Can you work these out from the model? Positions are in its coordinate system, mm. A direction names the side the tool comes from. Round coordinates to 2 decimals unless told otherwise and drop trailing zeros. Order: outer loops, then holes, each group sorted by start corner. A loop starts at its lowest first (then second) coordinate and runs counter-clockwise, first axis right, second up.
from build123d import *

# Parameters (mm, degrees)
SKETCH_1_R          = 1.5
EXTRUDE_1_DEPTH     = 3
SKETCH_2_R          = 1.5
CUT_EXTRUDE_1_DEPTH = 55.166410256
EXTRUDE_2_DEPTH     = 3
CUT_EXTRUDE_2_DEPTH = 55.166410256
CUT_EXTRUDE_3_DEPTH = 3
FILLET_1_R          = 3
EXTRUDE_3_DEPTH     = 3
FILLET_3_R          = 4
SKETCH_9_W          = 40
SKETCH_9_H          = 28
CUT_EXTRUDE_4_DEPTH = 10
FILLET_4_R          = 5
SKETCH_11_R         = 6.275308726
SKETCH_11_R_2       = 1.5
SKETCH_11_R_3       = 5.719245844
EXTRUDE_4_DEPTH     = 3
FILLET_5_R          = 30


with BuildPart() as part:
    # 草图1 → 凸台-拉伸1 (new body)
    with BuildSketch(Plane(origin=(0, 0, 0), x_dir=(1, 0, 0), z_dir=(0, 1, 0))):
        with BuildLine():
            Line((-17.5, -25), (-30, -25))
            Line((-30, -25), (-30, 25))
            Line((-30, 25), (-30, 29.606079858))
            ThreePointArc((-30, 29.606079858), (0, 25), (30, 29.606079858))
            Line((30, 29.606079858), (30, 25))
            Line((30, 25), (30, -25))
            Line((30, -25), (17.5, -25))
            Line((17.5, -25), (17.5, -45))
            Line((17.5, -45), (-17.5, -45))
            Line((-17.5, -45), (-17.5, -25))
        make_face()
        with Locations(Location((-14, -17, 0), (0, 0, 270))):
            Circle(SKETCH_1_R, mode=Mode.SUBTRACT)
        with Locations(Location((14, -17, 0), (0, 0, 90))):
            Circle(SKETCH_1_R, mode=Mode.SUBTRACT)
        with Locations(Location((-14, -28, 0), (0, 0, 270))):
            Circle(SKETCH_1_R, mode=Mode.SUBTRACT)
        with Locations(Location((14, -28, 0), (0, 0, 90))):
            Circle(SKETCH_1_R, mode=Mode.SUBTRACT)
        with BuildLine():
            Line((9.5, 20.5), (14.5, 20.5))
            ThreePointArc((14.5, 20.5), (16, 22), (14.5, 23.5))
            Line((14.5, 23.5), (9.5, 23.5))
            ThreePointArc((9.5, 23.5), (8, 22), (9.5, 20.5))
        make_face(mode=Mode.SUBTRACT)
        with BuildLine():
            Line((-2.5, 23.5), (2.5, 23.5))
            ThreePointArc((2.5, 23.5), (4, 22), (2.5, 20.5))
            Line((2.5, 20.5), (-2.5, 20.5))
            ThreePointArc((-2.5, 20.5), (-4, 22), (-2.5, 23.5))
        make_face(mode=Mode.SUBTRACT)
        with BuildLine():
            Line((-14.5, 23.5), (-9.5, 23.5))
            ThreePointArc((-9.5, 23.5), (-8, 22), (-9.5, 20.5))
            Line((-9.5, 20.5), (-14.5, 20.5))
            ThreePointArc((-14.5, 20.5), (-16, 22), (-14.5, 23.5))
        make_face(mode=Mode.SUBTRACT)
    extrude(amount=EXTRUDE_1_DEPTH)

    # 草图2 → 切除-拉伸1 (cut, through all)
    with BuildSketch(Plane(origin=(0, 3, 0), x_dir=(1, 0, 0), z_dir=(0, 1, 0))):
        with Locations(Location((-26, 19.5, 0), (0, 0, 270))):
            Circle(SKETCH_2_R)
        with Locations(Location((26, 19.5, 0), (0, 0, 90))):
            Circle(SKETCH_2_R)
        with BuildLine():
            Line((-6.4, 15.5), (-6.4, 0.5))
            ThreePointArc((-6.4, 0.5), (-10, -3.1), (-13.6, 0.5))
            Line((-13.6, 0.5), (-13.6, 15.5))
            ThreePointArc((-13.6, 15.5), (-10, 19.1), (-6.4, 15.5))
        make_face()
        with BuildLine():
            Line((6.4, 15.5), (6.4, 0.5))
            ThreePointArc((6.4, 0.5), (10, -3.1), (13.6, 0.5))
            Line((13.6, 0.5), (13.6, 15.5))
            ThreePointArc((13.6, 15.5), (10, 19.1), (6.4, 15.5))
        make_face()
    extrude(amount=-CUT_EXTRUDE_1_DEPTH, mode=Mode.SUBTRACT)

    # 草图3 → 凸台-拉伸2 (add)
    with BuildSketch(Plane(origin=(0, 3, 0), x_dir=(1, 0, 0), z_dir=(0, 1, 0))):
        Polygon((-30, -25), (-17.5, -45), (-17.5, -25), align=None)
        Polygon((17.5, -25), (17.5, -45), (30, -25), align=None)
    extrude(amount=-EXTRUDE_2_DEPTH)

    # 草图4 → 切除-拉伸2 (cut, through all)
    with BuildSketch(Plane(origin=(0, 3, 0), x_dir=(1, 0, 0), z_dir=(0, 1, 0))):
        Polygon((-30, 15), (-17.5, -45), (-30, -25), align=None)
        Polygon((17.5, -45), (30, -25), (30, 15), align=None)
    extrude(amount=-CUT_EXTRUDE_2_DEPTH, mode=Mode.SUBTRACT)

    # 草图6 → 切除-拉伸3 (cut)
    with BuildSketch(Plane(origin=(0, 3, 0), x_dir=(1, 0, 0), z_dir=(0, 1, 0))):
        Polygon((-10, -7), (10, -7), (7, -32), (-7, -32), align=None)
    extrude(amount=-CUT_EXTRUDE_3_DEPTH, mode=Mode.SUBTRACT)

    # 圆角1
    fillet_1_edges = [part.edges().sort_by_distance(p)[0] for p in [
        (10, 1.5, 7),
        (7, 1.5, 32),
        (-7, 1.5, 32),
        (-10, 1.5, 7),
    ]]
    fillet(fillet_1_edges, radius=FILLET_1_R)

    # 草图8 → 凸台-拉伸3 (add)
    with BuildSketch(Plane(origin=(0, 3, 0), x_dir=(1, 0, 0), z_dir=(0, 1, 0))):
        Polygon((-17.5, -45), (-17.083333333, -47), (17.083333333, -47), (17.5, -45), align=None)
    extrude(amount=-EXTRUDE_3_DEPTH)

    # 圆角3
    fillet_3_edges = [part.edges().sort_by_distance(p)[0] for p in [
        (-30, 1.5, -15),
        (30, 1.5, -15),
        (-30, 1.5, -29.606079858),
        (30, 1.5, -29.606079858),
        (17.083333333, 1.5, 47),
        (-17.083333333, 1.5, 47),
    ]]
    fillet(fillet_3_edges, radius=FILLET_3_R)

    # 草图9 → 切除-拉伸4 (cut)
    with BuildSketch(Plane(origin=(0, 3, 0), x_dir=(1, 0, 0), z_dir=(0, 1, 0))):
        with Locations((0, -47)):
            Rectangle(SKETCH_9_W, SKETCH_9_H)
    extrude(amount=-CUT_EXTRUDE_4_DEPTH, mode=Mode.SUBTRACT)

    # 圆角4
    fillet_4_edges = [part.edges().sort_by_distance(p)[0] for p in [
        (-20, 1.5, 33),
        (20, 1.5, 33),
    ]]
    fillet(fillet_4_edges, radius=FILLET_4_R)

    # 草图11 → 凸台-拉伸4 (add)
    # profile 1 of 2: a face of its own
    with BuildSketch(Plane(origin=(0, 3, 0), x_dir=(1, 0, 0), z_dir=(0, 1, 0))):
        with Locations((-26, 19.5)):
            Circle(SKETCH_11_R)
        with Locations(Location((-26, 19.5, 0), (0, 0, 270))):
            Circle(SKETCH_11_R_2, mode=Mode.SUBTRACT)
    # profile 2 of 2: a face of its own
    with BuildSketch(Plane(origin=(0, 3, 0), x_dir=(1, 0, 0), z_dir=(0, 1, 0))):
        with Locations((26, 19.5)):
            Circle(SKETCH_11_R_3)
        with Locations(Location((26, 19.5, 0), (0, 0, 90))):
            Circle(SKETCH_11_R_2, mode=Mode.SUBTRACT)
    extrude(amount=-EXTRUDE_4_DEPTH)

    # 圆角5
    fillet_5_edges = [part.edges().sort_by_distance(p)[0] for p in [
        (30, 1.5, -15.412241075),
        (30, 1.5, -23.587758925),
        (-29.915921679, 1.5, -14.596424059),
        (-29.999864579, 1.5, -24.335347242),
    ]]
    fillet(fillet_5_edges, radius=FILLET_5_R)


solid = part.part
(1) If we mould it in two halves opening along X, with no side actions, what happens to faces 1 (the face through (-19.126, 1.479, 31.849)), 2 (the face through (-16, 1, -22)), 3 (the face through (19.05, 1.48, 31.91))? For each: pulls with the +X half, pulls with the -X half, needs draft (parallel to the pull), parting line crosses it, or undercut.
(2) I want a section at B-B, the plane z = 17.5. List the corners of the cut face in (x, y) for me.
(3) Please list where these lines run through material, in increasing order: probe 1 along Z at (x, y) = (14, 2.1); probe 2 along X at (y, z) = (1.7, -19.5); probe 3 along Z at (x, y) = (-1.5, 0.4).
(4) I want a section at D-D, the plane y = 0.9. Give the number of separate pieces and of enclosed holes in the cut face, plus the area to 3 significant figures.
(5) On a 3-axis mill with a long thin cutter (end or side, diameter ignored), from which of +Z, -Z, +X, -X, +Y, -Y can I reach the whole of each face in a straight line? I mean faces 4 (the face through (-27.75, 1.52, -27.9)), 5 (the face through (6.31, 1.48, 31.26)). Say none if no direction works.
(6) I want a section at C-C, the plane z = 9. List the corners of the cut face in (x, y) for me.
(7) I'm going to push a flat-ended pin straight in: pin 1 Ø1.5 at (y, z) = (2, -8.5) entering from +X. Where does the tip first touch, or does it pass through?
(8) I want a section at A-A, the plane z = 1. List the corners of the cut face in (x, y) for me, plus the area to 3 significant figures.
Ans:
1. face 1: pulls with the -X half
1. face 2: undercut
1. face 3: pulls with the +X half
2. outline: (-23.23, 0) - (-15.41, 0) - (-15.41, 3) - (-23.23, 3) - close; (-12.59, 0) - (-8.74, 0) - (-8.74, 3) - (-12.59, 3) - close; (8.74, 0) - (12.59, 0) - (12.59, 3) - (8.74, 3) - close; (15.41, 0) - (23.23, 0) - (23.23, 3) - (15.41, 3) - close
3. probe 1: z = -25.98 to -23.5, -20.5 to 15.5, 18.5 to 26.5, 29.5 to 33
3. probe 2: x = -32.28 to -27.5, -24.5 to 24.5, 27.5 to 31.72
3. probe 3: z = -25.01 to -23.5, -20.5 to 7, 32 to 33
4. separate pieces: 1
4. enclosed holes: 12
4. area: 2,280 mm2
5. face 4: -Z, +Y, -Y
5. face 5: +Y, -Y
6. outline: (-25, 0) - (-9.45, 0) - (-9.45, 3) - (-25, 3) - close; (9.45, 0) - (25, 0) - (25, 3) - (9.45, 3) - close
7. pin 1: stops at x = 28.8
8. outline: (-26.67, 0) - (-13.27, 0) - (-13.27, 3) - (-26.67, 3) - close; (-6.73, 0) - (6.73, 0) - (6.73, 3) - (-6.73, 3) - close; (13.27, 0) - (26.67, 0) - (26.67, 3) - (13.27, 3) - close
8. area: 121 mm2
